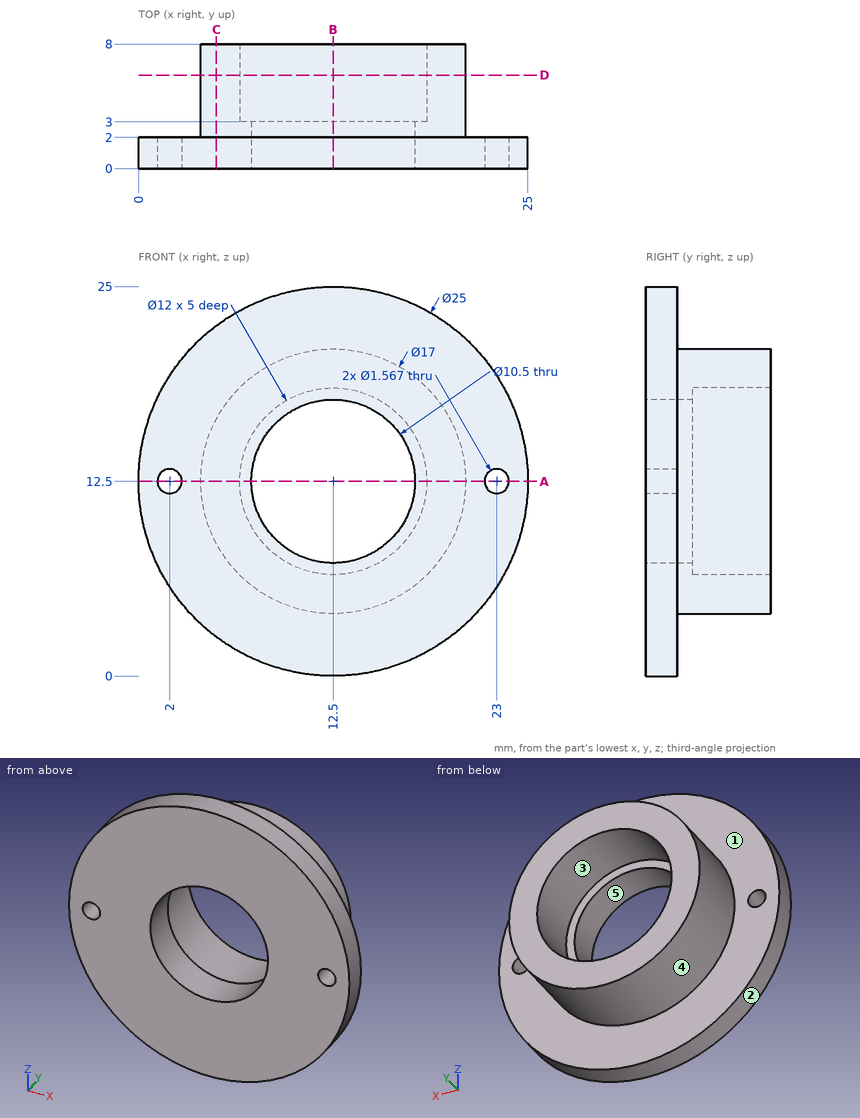
Geometry check sheet. Reference: drawing and pictorial views, mm from the part's lowest x, y, z. A direction names the side the tool comes from. Round coordinates to 2 decimals unless told otherwise and drop trailing zeros. Write each loop counter-clockwise with the first axis right and the second up, starting at its lowest first coordinate (ties: lowest second). Pieces come first, ordered by that corner, then holes. Notation, with made-up numbers: (-33, -34.75) -> (-5, -34.75) arc R32 ccw to (-5, 2.25) -> close; hole circle Ø5 at (46, 82.25). An arc over 180 degrees is marked (long way). Put each result on its own line as item: value.
1) Access from +Z, -Z, +X, -X, +Y, -Y to the whole of each face (thin tool, end or side, straight path). Record for the marked faces 4 and 5.
Recorded:
face 4: +Y
face 5: +Y, -Y
2) Cross-section at C-C, the plane x = 5. Enter the section's corners in (y, z).
Recorded:
outline: (0, 2.5) -> (2, 2.5) -> (2, 8.5) -> (8, 8.5) -> (8, 16.5) -> (2, 16.5) -> (2, 22.5) -> (0, 22.5) -> close
3) Thickness scan on probe 1 along X at (y, z) = (1, 12.5); probe 2 along X at (y, z) = (5.15, 12.5); probe 3 along Z at (x, y) = (12.75, 6). Record the ranges inside material, lowest first. Write a range as from..to.
Recorded:
probe 1: x = 0..1.22, 2.78..7.25, 17.75..22.22, 23.78..25
probe 2: x = 4..6.5, 18.5..21
probe 3: z = 4..6.51, 18.49..21
4) Cross-section at D-D, the plane y = 6. Enter the section's corners in (x, z).
Recorded:
outline: circle Ø17 at (12.5, 12.5); hole circle Ø12 at (12.5, 12.5)
5) Depth check by flat-ended pin: P1, Ø6, axis at x = 11, z = 15, coming from the +Y side; P2, Ø4, axis at x = 15, y = 1.5, coming from the -Z side; P3, Ø2, axis at x = 16, y = 2, coming from the -Z side; P4, Ø1.3, axis at x = 23, z = 12.5, coming from the -Y side. Enter the tip coordinate at first touch or a pass-through.
Recorded:
P1: stops at y = 3
P2: stops at z = 0.01
P3: stops at z = 0.25
P4: passes through
6) Cross-section at A-A, the plane z = 12.5. Enter the section's corners in (x, y).
Recorded:
outline: (0, 0) -> (1.22, 0) -> (1.22, 2) -> (0, 2) -> close; (2.78, 0) -> (7.25, 0) -> (7.25, 3) -> (6.5, 3) -> (6.5, 8) -> (4, 8) -> (4, 2) -> (2.78, 2) -> close; (17.75, 0) -> (22.22, 0) -> (22.22, 2) -> (21, 2) -> (21, 8) -> (18.5, 8) -> (18.5, 3) -> (17.75, 3) -> close; (23.78, 0) -> (25, 0) -> (25, 2) -> (23.78, 2) -> close
7) Release check for a two-part mould opening along Z. For the marked faces 1, 2 and 3 record: pulls with the +Z half, pulls with the -Z half, needs draft (parallel to the pull), parting line crosses it, or undercut.
Recorded:
face 1: needs draft
face 2: parting line crosses it
face 3: undercut
8) Cross-section at B-B, the plane x = 12.5. Enter the section's corners in (y, z).
Recorded:
outline: (0, 0) -> (2, 0) -> (2, 4) -> (8, 4) -> (8, 6.5) -> (3, 6.5) -> (3, 7.25) -> (0, 7.25) -> close; (0, 17.75) -> (3, 17.75) -> (3, 18.5) -> (8, 18.5) -> (8, 21) -> (2, 21) -> (2, 25) -> (0, 25) -> close
